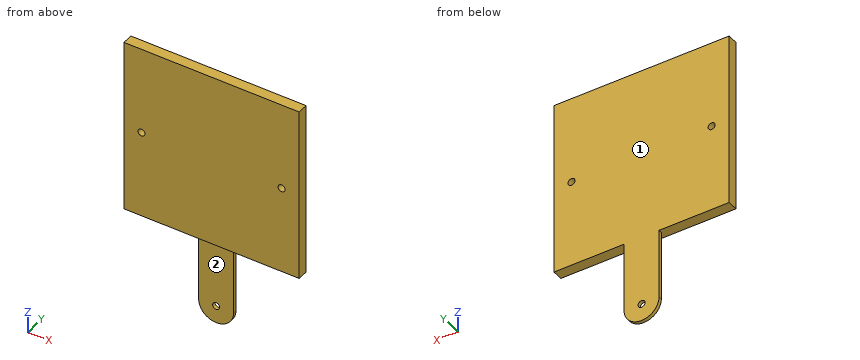
```python
from build123d import *

# Parameters (mm, degrees)
SKETCH1_R           = 10
BOSS_EXTRUDE1_DEPTH = 10
SKETCH2_W           = 500
SKETCH2_H           = 500
BOSS_EXTRUDE2_DEPTH = 20
SKETCH3_R           = 10
CUT_EXTRUDE1_DEPTH  = 744.908596536


with BuildPart() as part:
    # Sketch1 → Boss-Extrude1 (new body)
    with BuildSketch(Plane(origin=(0, 0, 0), x_dir=(1, 0, 0), z_dir=(0, 1, 0))):
        with BuildLine():
            Line((-50, 0), (-50, -200))
            Line((-50, -200), (-250, -200))
            Line((-250, -200), (-250, -700))
            Line((-250, -700), (250, -700))
            Line((250, -700), (250, -200))
            Line((250, -200), (50, -200))
            Line((50, -200), (50, 0))
            ThreePointArc((50, 0), (0, 50), (-50, 0))
        make_face()
        with Locations(Location((0, 0, 0), (0, 0, 270))):
            Circle(SKETCH1_R, mode=Mode.SUBTRACT)
    extrude(amount=BOSS_EXTRUDE1_DEPTH)

    # Sketch2 → Boss-Extrude2 (add)
    with BuildSketch(Plane.XZ):
        with Locations((0, 450)):
            Rectangle(SKETCH2_W, SKETCH2_H)
    extrude(amount=BOSS_EXTRUDE2_DEPTH)

    # Sketch3 → Cut-Extrude1 (cut, through all)
    with BuildSketch(Plane(origin=(0, 10, 0), x_dir=(1, 0, 0), z_dir=(0, 1, 0))):
        with Locations(Location((200, -450, 0), (0, 0, 270))):
            Circle(SKETCH3_R)
        with Locations(Location((-200, -450, 0), (0, 0, 90))):
            Circle(SKETCH3_R)
    extrude(amount=-CUT_EXTRUDE1_DEPTH, mode=Mode.SUBTRACT)


solid = part.part
```
Read the model definition and answer for the solid it produces. Units are mm, in the model's axes. Face numbers are marked on the shaded views. A direction names the side the tool comes from. Coordinates: 2 decimals unless noted, no trailing zeros. Write each loop counter-clockwise with the first axis right and the second up, starting at its lowest first coordinate (ties: lowest second). Pieces come first, ordered by that corner, then holes. Notation, with made-up numbers: (9.25, 59) - (38.25, 59) arc R23 cw to (38.25, 70) - close; hole circle Ø5 at (-7, -6.75). An arc over 180 degrees is marked (long way). Answer as a JSON object with one key per item and string values. Group by question number.
1. A cutting plane is placed at C-C (y = -8). Determine the outline of the cut face in (x, z).
2. A cutting plane is placed at D-D (x = 0). Determine the outline of the cut face in (y, z).
3. A cutting plane is placed at A-A (z = 450). Determine the outline of the cut face in (x, y), plus the area to 3 significant figures.
4. Each of these flat-tipped pins is pushed along its axis until it touches: P1, Ø8, axis at x = -7, y = 3, coming from the -Z side; P2, Ø8, axis at y = 3.5, z = 66.5, coming from the -X side; P3, Ø8, axis at x = 66.5, y = -4, coming from the -Z side. Where does it stop, or does it pass through?
5. Which of the six approach directions +Z, -Z, +X, -X, +Y, -Y give full straight-line access (tool end or side, diameter ignored) to the marked faces 1 and 2?
6. A cutting plane is placed at B-B (x = -200). Determine the outline of the cut face in (y, z), plus the area to 3 significant figures.
7. Consider L1, parallel to X at y = -3.5, z = 450; L2, parallel to Z at x = -200, y = -3.75; L3, parallel to Z at x = -32.5, y = -2.75. Determine where each line is inside the solid, lowest interval first. Write a range as [from, to].
Worked out:
{
 "1": {"outline": "(-250, 200) - (250, 200) - (250, 700) - (-250, 700) - close; hole circle Ø20 at (-200, 450); hole circle Ø20 at (200, 450)"},
 "2": {"outline": "(-20, 200) - (0, 200) - (0, 10) - (10, 10) - (10, 700) - (-20, 700) - close; (0, -50) - (10, -50) - (10, -10) - (0, -10) - close"},
 "3": {"outline": "(-250, -20) - (-210, -20) - (-210, 10) - (-250, 10) - close; (-190, -20) - (190, -20) - (190, 10) - (-190, 10) - close; (210, -20) - (250, -20) - (250, 10) - (210, 10) - close", "area": "13,800 mm²"},
 "4": {"P1": "stops at z = -49.91", "P2": "stops at x = -50", "P3": "stops at z = 200"},
 "5": {"face 1": "+Z, -Z, +X, -X, +Y", "face 2": "-Z, +X, -X, -Y"},
 "6": {"outline": "(-20, 200) - (10, 200) - (10, 440) - (-20, 440) - close; (-20, 460) - (10, 460) - (10, 700) - (-20, 700) - close", "area": "14,400 mm²"},
 "7": {"L1": "x = [-250, -210], [-190, 190], [210, 250]", "L2": "z = [200, 440], [460, 700]", "L3": "z = [200, 700]"}
}
